Geometry check sheet. Reference: the model listing, model coordinates, mm. Face numbers are marked on the shaded views. A direction names the side the tool comes from. Give positions to 0.01 mm unless a question says otherwise; leave off trailing zeros. Order: outer loops, then holes, each group sorted by start corner. A loop starts at its lowest first (then second) coordinate and runs counter-clockwise, first axis right, second up. Notation, with made-up numbers: M 47.5,-17 L 101.5,-17 A25 ccw 101.5,10 Z; hole C -39,38.25 d10. An arc over 180 degrees is marked long. Answer as CSV lines item,"result". Start each with the question number.
Q1. Go/stop test with flat-tipped pins: pin 1 (4 mm diameter, centred on x = -65, z = -2.5, fed in from +Y); pin 2 (0.9 mm diameter, centred on y = 16, z = 38.5, fed in from -X); pin 3 (9 mm diameter, centred on x = 52.5, z = 6.5, fed in from -Y); pin 4 (6.5 mm diameter, centred on x = -65, z = 27.5, fed in from -Y). Record where each tip stops, or that it passes through.
Q2. Thickness scan on line 1 (Z direction, x = -20, y = 6.25); line 2 (X direction, y = 6.75, z = 6.5); line 3 (Z direction, x = -77, y = 12.5). Record the ranges inside material, lowest first.
Q3. Section check C-C, the plane x = 54. Record the boundary of the cut face in (y, z), then the cut area to 3 significant figures.
Q4. Section check A-A, the plane z = 66.5. Record the boundary of the cut face in (x, y), then the cut area to 3 significant figures.
Q5. Set-up check for the marked faces 1, 2 and 3: record each of +Z, -Z, +X, -X, +Y, -Y from which the full face is reachable in a straight line by a thin tool's end or side.
Q6. Section check B-B, the plane x = -75.5. Record the boundary of the cut face in (y, z), then the cut area to 3 significant figures.
Q7. Section check D-D, the plane y = 9.5. Count the separate pieces of the cut face and the enclosed holes in it, then the cut area to 3 significant figures.
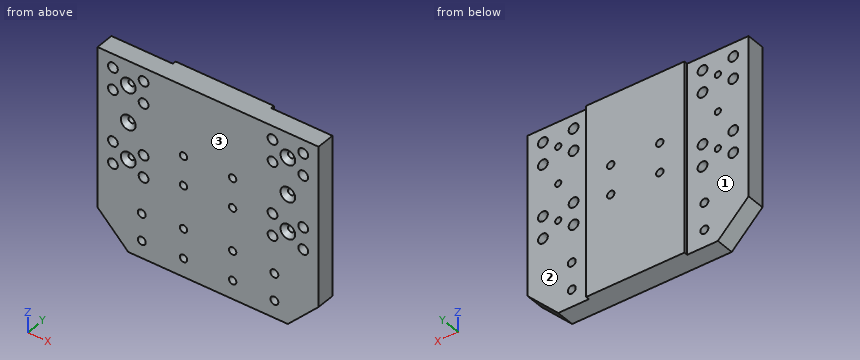
Autodesk Fusion 360 part; units mm, degrees
sketch "Spindle Mount Board" plane through (0, 0, 0) normal (0, 1, 0) x (1, 0, 0)
  line L0 (90, -77.5) -> (-90, -77.5) construction
  line L1 (-90, -77.5) -> (-90, 52.5) construction
  line L2 (-65, 77.5) -> (65, 77.5) construction
  line L3 (90, 52.5) -> (90, -77.5) construction
  line L4 (90, -77.5) -> (-90, 77.5) construction
  line L5 (-90, -77.5) -> (90, 77.5) construction
  line L6 (-90, -77.5) -> (90, -77.5)
  line L7 (90, -77.5) -> (90, 52.5)
  line L8 (90, 52.5) -> (65, 77.5)
  line L9 (90, 52.5) -> (125.7504, 52.5) construction
  line L10 (-90, -77.5) -> (-90, 52.5)
  line L11 (-90, 52.5) -> (-65, 77.5)
  line L12 (-90, 52.5) -> (-54.1427, 52.5) construction
  line L13 (-65, 77.5) -> (65, 77.5)
  line L14 (-77.5, -77.5) -> (-77.5, 25) construction
  line L15 (-52.5, -77.5) -> (-52.5, 25) construction
  line L16 (77.5, -77.5) -> (77.5, 25) construction
  line L17 (52.5, -77.5) -> (52.5, 25) construction
  line L18 (-90, -66.5) -> (90, -66.5) construction
  line L19 (-90, -48.5) -> (90, -48.5) construction
  line L20 (-90, -6.5) -> (90, -6.5) construction
  line L21 (-90, 11.5) -> (90, 11.5) construction
  circle A0 centre (-77.5, -66.5) radius 4
  circle A1 centre (77.5, -66.5) radius 4
  circle A2 centre (-52.5, -66.5) radius 4
  circle A3 centre (52.5, -66.5) radius 4
  circle A4 centre (-77.5, -48.5) radius 4
  circle A5 centre (-52.5, -48.5) radius 4
  circle A6 centre (52.5, -48.5) radius 4
  circle A7 centre (77.5, -48.5) radius 4
  circle A8 centre (-77.5, -6.5) radius 4
  circle A9 centre (-52.5, -6.5) radius 4
  circle A10 centre (52.5, -6.5) radius 4
  circle A11 centre (77.5, -6.5) radius 4
  circle A12 centre (-77.5, 11.5) radius 4
  circle A13 centre (-52.5, 11.5) radius 4
  circle A14 centre (52.5, 11.5) radius 4
  circle A15 centre (77.5, 11.5) radius 4
  line L22 (65, -77.5) -> (65, 25) construction
  line L23 (-65, -77.5) -> (-65, 25) construction
  line L24 (-70, -57.5) -> (70, -57.5) construction
  line L25 (-70, -27.5) -> (70, -27.5) construction
  line L26 (-70, 2.5) -> (70, 2.5) construction
  circle A16 centre (-65, -57.5) radius 2.5
  circle A17 centre (-65, -27.5) radius 2.5
  circle A18 centre (-65, 2.5) radius 2.5
  circle A19 centre (65, 2.5) radius 2.5
  circle A20 centre (65, -27.5) radius 2.5
  circle A21 centre (65, -57.5) radius 2.5
  line L27 (-54, 41.5) -> (54, 41.5) construction
  line L28 (54, 41.5) -> (54, 63.5) construction
  line L29 (54, 63.5) -> (-54, 63.5) construction
  line L30 (-54, 63.5) -> (-54, 41.5) construction
  circle A22 centre (-54, 41.5) radius 3.25
  circle A23 centre (-54, 63.5) radius 3.25
  circle A24 centre (54, 41.5) radius 3.25
  circle A25 centre (54, 63.5) radius 3.25
  line L31 (-20, -20.5) -> (20, -20.5) construction
  line L32 (20, -20.5) -> (20, 3.5) construction
  line L33 (20, 3.5) -> (-20, 3.5) construction
  line L34 (-20, 3.5) -> (-20, -20.5) construction
  circle A26 centre (-20, -20.5) radius 3
  circle A27 centre (-20, 3.5) radius 3
  circle A28 centre (20, -20.5) radius 3
  circle A29 centre (20, 3.5) radius 3
  line L35 (-90, -77.5) -> (-40, -77.5)
  line L36 (-40, -77.5) -> (-40, 77.5)
  line L37 (-40, 77.5) -> (-65, 77.5)
  line L38 (-90, 52.5) -> (-90, -77.5)
  line L39 (90, -77.5) -> (40, -77.5)
  line L40 (40, -77.5) -> (40, 77.5)
  line L41 (40, 77.5) -> (65, 77.5)
  line L42 (90, 52.5) -> (90, -77.5)
  line L43 (-20, 38.5) -> (20, 38.5) construction
  line L44 (20, 38.5) -> (20, 62.5) construction
  line L45 (20, 62.5) -> (-20, 62.5) construction
  line L46 (-20, 62.5) -> (-20, 38.5) construction
  circle A30 centre (-20, 38.5) radius 3
  circle A31 centre (20, 38.5) radius 3
  circle A32 centre (-20, 62.5) radius 3
  circle A33 centre (20, 62.5) radius 3
  dimension "d1" = 180
  dimension "d2" = 155
  dimension "d3" = 130
  dimension "d4" = 135
  dimension "d5" = 130
  dimension "d6" = 45
  dimension "d7" = 25
  dimension "d8" = 25
  dimension "d9" = 25
  dimension "d10" = 25
  dimension "d11" = 12.5
  dimension "d12" = 12.5
  dimension "d13" = 25
  dimension "d14" = 25
  dimension "d15" = 11
  dimension "d16" = 18
  dimension "d17" = 18
  dimension "d18" = 42
  dimension "d19" = 8
  dimension "d20" = 8
  dimension "d21" = 8
  dimension "d22" = 8
  dimension "d23" = 8
  dimension "d24" = 8
  dimension "d25" = 8
  dimension "d26" = 8
  dimension "d27" = 8
  dimension "d28" = 8
  dimension "d29" = 8
  dimension "d30" = 8
  dimension "d31" = 8
  dimension "d32" = 8
  dimension "d33" = 8
  dimension "d34" = 8
  dimension "d35" = 25
  dimension "d36" = 25
  dimension "d37" = 30
  dimension "d38" = 30
  dimension "d39" = 20
  dimension "d40" = 5
  dimension "d41" = 5
  dimension "d42" = 5
  dimension "d43" = 5
  dimension "d44" = 5
  dimension "d45" = 5
  dimension "d46" = 108
  dimension "d47" = 22
  dimension "d48" = 54
  dimension "d49" = 14
  dimension "d50" = 6.5
  dimension "d51" = 6.5
  dimension "d52" = 6.5
  dimension "d53" = 6.5
  dimension "d54" = 24
  dimension "d55" = 20
  dimension "d56" = 57
  dimension "d57" = 6
  dimension "d58" = 6
  dimension "d59" = 6
  dimension "d60" = 6
  dimension "d61" = 50
  dimension "d62" = 50
  dimension "d67" = 40
  dimension "d68" = 24
  dimension "d69" = 20
  dimension "d70" = 3
  dimension "d71" = 6
  dimension "d72" = 6
  dimension "d73" = 6
  dimension "d74" = 6
extrude "Extrude3" add sketch "Spindle Mount Board" along normal blind 18 contours L6 L13 L36 L40
extrude "Extrude4" add sketch "Spindle Mount Board" along normal blind 15 contours L6 L10 L11 L13 L35 L36 L37 L38 | L6 L7 L8 L13 L39 L40 L41 L42
extrude "Extrude5" add sketch "Spindle Mount Board" along normal blind 18 contours A30 | A31 | A32 | A33
extrude "Extrude6" cut sketch "Spindle Mount Board" along normal blind 6 contours A30 | A31 | A32 | A33
chamfer "Chamfer1" distance 3.5 angle 45 6 edges at (-67.3308, 0, 56.596) (-67.3308, 0, 26.596) (-67.3308, 0, -3.404) (62.6692, 0, -3.404) (62.6692, 0, 26.596) (62.6692, 0, 56.596)
Answer block:
1,pin 1,"passes through"
1,pin 2,"stops at x = -40"
1,pin 3,"stops at y = 0"
1,pin 4,"stops at y = 2.75"
2,line 1,"z = -77.5 to -6.5, -0.5 to 17.5, 23.5 to 77.5"
2,line 2,"x = -90 to -81.5, -73.5 to -56.5, -48.5 to 48.5, 56.5 to 73.5, 81.5 to 90"
2,line 3,"z = -65.5 to -15.47, -7.53 to 2.53, 10.47 to 44.53, 52.47 to 62.53, 70.47 to 77.5"
3,outline,"M 0,-77.5 L 15,-77.5 L 15,-66.75 L 0,-66.75 Z; M 0,-60.25 L 15,-60.25 L 15,-44.75 L 0,-44.75 Z; M 0,-38.25 L 15,-38.25 L 15,-15.21 L 0,-15.21 Z; M 0,-7.79 L 15,-7.79 L 15,2.79 L 0,2.79 Z; M 0,10.21 L 15,10.21 L 15,44.79 L 0,44.79 Z; M 0,52.21 L 15,52.21 L 15,62.79 L 0,62.79 Z; M 0,70.21 L 15,70.21 L 15,77.5 L 0,77.5 Z"
3,area,"1,690 mm2"
4,outline,"M -90,0 L -81.5,0 L -81.5,15 L -90,15 Z; M -73.5,0 L -56.5,0 L -56.5,15 L -73.5,15 Z; M -48.5,0 L 48.5,0 L 48.5,15 L 40,15 L 40,18 L -40,18 L -40,15 L -48.5,15 Z; M 56.5,0 L 73.5,0 L 73.5,15 L 56.5,15 Z; M 81.5,0 L 90,0 L 90,15 L 81.5,15 Z"
4,area,"2,460 mm2"
5,face 1,"+Z, -Z, -X, +Y"
5,face 2,"+Z, -Z, +X, +Y"
5,face 3,"+Z, -Z, +X, -X, -Y"
6,outline,"M 0,-67 L 15,-67 L 15,-14.96 L 0,-14.96 Z; M 0,-8.04 L 15,-8.04 L 15,3.04 L 0,3.04 Z; M 0,9.96 L 15,9.96 L 15,45.04 L 0,45.04 Z; M 0,51.96 L 15,51.96 L 15,63.04 L 0,63.04 Z; M 0,69.96 L 15,69.96 L 15,77.5 L 0,77.5 Z"
6,area,"1,750 mm2"
7,separate pieces,"1"
7,enclosed holes,"30"
7,area,"26,100 mm2"
